Verification items for the finished model (mm, model axes). A direction names the side the tool comes from. Coordinates: 2 decimals unless noted, no trailing zeros. Write each loop counter-clockwise with the first axis right and the second up, starting at its lowest first coordinate (ties: lowest second). Pieces come first, ordered by that corner, then holes. Notation, with made-up numbers: M 17.5,-7 L 43.5,-7 A30 ccw 43.5,15 Z; hole C 40,81 d11. An arc over 180 degrees is marked long. Answer in a Markdown table with one row per item.
from build123d import *

# Parameters (mm, degrees)
F0_R     = 15.9004
F1_DEPTH = 7.239
F2_R     = 1.89865
F3_DEPTH = 14.479
F6_W     = 3.175
F6_H     = 7.507812879


# Not quite as in the source:
# - a feature names something its author has since deleted; it is built from what else it names


with BuildPart() as f1:
    # F0 (on Top) → F1 (new body, symmetric)
    with BuildSketch(Plane.XY):
        Circle(F0_R)
    extrude(amount=F1_DEPTH, both=True)

    # F2 (on face) → F3 (cut, through all)
    with BuildSketch(Plane.XY.offset(7.239)):
        Circle(F2_R)
    extrude(amount=-F3_DEPTH, mode=Mode.SUBTRACT)

    # F4 (on Right) → F5 (revolve, cut)
    with BuildSketch(Plane.YZ):
        Polygon((18.6176884613, -4.7117), (18.6176884613, 4.7117), (12.3317, 4.7117), (7.62, 0), (12.3317, -4.7117), align=None)
        Polygon((5.715, 2.5851280605), (12.0073856063, 8.8775136668), (5.715, 8.8775136668), align=None)
    revolve(axis=Axis((0, 0, 8.1515284255), (0, 0, 1)), mode=Mode.SUBTRACT)

    # F6 (on face) → F7 (join, up to the next surface of F1)
    with BuildSketch(Plane.XY.offset(7.239)):
        with Locations((0, 7.7054322143)):
            Rectangle(F6_W, F6_H)
        Polygon((-10.4079142205, 5.0509326079), (-11.3890431777, 2.0313281687), (-4.248688816, -0.2887136015), (-3.2675598588, 2.7308908377), align=None)
        Polygon((-8.0199447403, -8.3376906272), (-5.4513157831, -10.2039088032), (-1.0383340959, -4.1299605935), (-3.606963053, -2.2637424175), align=None)
        Polygon((5.4513157831, -10.2039088032), (8.0199447403, -8.3376906272), (3.606963053, -2.2637424175), (1.0383340959, -4.1299605935), align=None)
        Polygon((11.3890431777, 2.0313281687), (10.4079142205, 5.0509326079), (3.2675598588, 2.7308908377), (4.248688816, -0.2887136015), align=None)
    extrude(until=Until.NEXT, dir=(0, 0, -1))


solid = f1.part
1) Sectioned sample at A-A (x = 0). Record the cut outline in (y, z) (3 decimals).
Response values:
| item | result |
|---|---|
| outline | M -15.9,-7.239 L -1.899,-7.239 L -1.899,7.239 L -5.715,7.239 L -5.715,2.585 L -10.369,7.239 L -15.9,7.239 L -15.9,4.712 L -12.332,4.712 L -7.62,0 L -12.332,-4.712 L -15.9,-4.712 Z; M 1.899,-7.239 L 15.9,-7.239 L 15.9,-4.712 L 12.332,-4.712 L 7.62,0 L 12.332,4.712 L 15.9,4.712 L 15.9,7.239 L 1.899,7.239 Z |
2) Depth check by flat-ended pin: pin 1 (1 mm diameter, centred on y = 10.5, z = -4, fed in from +X); pin 2 (1.4 mm diameter, centred on y = 7, z = 4.5, fed in from -X); pin 3 (1 mm diameter, centred on x = 4, z = -2, fed in from +Y). Enter the tip coordinate at first touch or a pass-through.
Response values:
| item | result |
|---|---|
| pin 1 | stops at x = 6.36 |
| pin 2 | stops at x = -14.58 |
| pin 3 | stops at y = 9.34 |
3) Sectioned sample at C-C (z = 6.25). Record the cut outline in (x, y) (1 decimal), then the cut area to 3 significant figures.
Response values:
| item | result |
|---|---|
| outline | C 0,0 d31.8; hole M -9.3,1.3 A9.4 ccw -6.7,-6.5 L -4.5,-3.5 A5.7 cw -5.7,0.2 Z; hole M -8.3,4.4 L -4.7,3.2 A5.7 cw -1.6,5.5 L -1.6,9.2 A9.4 ccw Z; hole M -4.1,-8.4 A9.4 ccw 4.1,-8.4 L 1.9,-5.4 A5.7 cw -1.9,-5.4 Z; hole C 0,0 d3.8; hole M 1.6,5.5 A5.7 cw 4.7,3.2 L 8.3,4.4 A9.4 ccw 1.6,9.2 Z; hole M 4.5,-3.5 L 6.7,-6.5 A9.4 ccw 9.3,1.3 L 5.7,0.2 A5.7 cw Z |
| area | 668 mm² |
4) Sectioned sample at B-B (y = -13). Record the cut outline in (x, z).
Response values:
| item | result |
|---|---|
| outline | M -9.16,-7.24 L 9.16,-7.24 L 9.16,-4.71 L -9.16,-4.71 Z; M -9.16,4.71 L 9.16,4.71 L 9.16,7.24 L -9.16,7.24 Z |
5) Thickness scan on L1, parallel to Z at x = 9.5, y = -9; L2, parallel to Y at x = 1, z = 6.75; L3, parallel to Z at x = -4.5, y = -9. Record the ranges inside material, lowest first. Write a range as [from, to].
Response values:
| item | result |
|---|---|
| L1 | z = [-7.24, -4.71], [4.71, 7.24] |
| L2 | y = [-15.87, -9.83], [-5.63, -1.61], [1.61, 15.87] |
| L3 | z = [-7.24, -2.44], [2.44, 6.93] |
6) Tool access check on faces 1 (the face through (5.618, -5.032, 5.462)), 2 (the face through (-2.358, 7.486, 0.229)), 3 (the face through (-3.45, -15.52, 5.99)). Record the directions out of +Z, -Z, +X, -X, +Y, -Y that give a thin tool (end or side, any length) a straight path to the whole face; none if there is none.
Response values:
| item | result |
|---|---|
| face 1 | +Z |
| face 2 | none |
| face 3 | +Z, -Z |
7) Release check for a two-part mould opening along Z. For faces 4 (the face through (0, -3, 7.239)), 5 (the face through (0, -3, -7.239)), 6 (the face through (12, 5, 4.712)), 7 (the face through (-7.503, 0.769, 5.462)) record: +Z half, -Z half, draft (parallel to the pull), parting line (faces both ways), or undercut.
Response values:
| item | result |
|---|---|
| face 4 | +Z half |
| face 5 | -Z half |
| face 6 | undercut |
| face 7 | draft |
8) Sectioned sample at D-D (z = 2). Record the cut outline in (x, y).
Response values:
| item | result |
|---|---|
| outline | C 0,0 d19.24; hole C 0,0 d3.8 |
